Check sheet for the modelled part. Datum: model origin and axes. Units: mm. A direction names the side the tool comes from. Give positions to 0.01 mm unless a question says otherwise; leave off trailing zeros. Loops run counter-clockwise (first coordinate to the right, second up) from the corner with the lowest first, then second, coordinate; pieces in that order, holes last. Notation, with made-up numbers: (39.5, 12) -> (50.5, 12) arc R22 ccw to (50.5, 45) -> close; hole circle Ø2 at (32.25, 12). An arc over 180 degrees is marked (long way). Write each question's results on one line, items separated by ' | '. Start each with the question number.
1. Material ranges on L1, parallel to Z at x = 0, y = 29.5; L2, parallel to X at y = 36.5, z = -9.1; L3, parallel to Y at x = -0.35, z = -7.4, recorded low to high. Write a range as from..to.
2. Cross-section at B-B on y = 13. Record the boundary of the cut face in (x, z).
3. Gauge pin test, flat end, axial feed: pin 1 Ø0.8 at (x, z) = (0, -9) entering from -Y. Record the tip position at first contact, or that the pin passes through.
4. Tool access check on faces 5 (the face through (-0.011, 40.364, -5.496)), 6 (the face through (-0.104, 33.549, -9.793)). Record the directions out of +Z, -Z, +X, -X, +Y, -Y that give a thin tool (end or side, any length) a straight path to the whole face; none if there is none.
5. Cross-section at A-A on x = 0. Record the boundary of the cut face in (y, z), and give its area (3 significant figures).
6. Mould release check, pull along Y, two halves, no side actions. Record for faces 1 (the face through (-0.104, 12.591, -9.793)), 2 (the face through (0.43, 40.735, -6.483)), 3 (the face through (0.098, 24.423, -8.256)), 4 (the face through (-0.12, 2.96, -9.89)): +Y half, -Y half, draft (parallel to the pull), parting line (faces both ways), or undercut.
from build123d import *

# Parameters (mm, degrees)
SKETCH2_R         = 0.8
SKETCH4_R         = 0.9
EXTRUDE1_DEPTH    = 6
SKETCH5_OUTSIDE_W = 12.086
SKETCH5_OUTSIDE_H = 14.96
SKETCH5_OUTSIDE_R = 0.75
EXTRUDE3_DEPTH    = 11


with BuildPart() as part:
    # Sweep1: sweep along a path in Sketch1
    with BuildLine(Plane(origin=(0, 0, 0), x_dir=(0, 0, -1), z_dir=(1, 0, 0))) as sweep1_path:
        Line((9, 0), (9, 37))
        ThreePointArc((9, 37), (8.457456133, 38.720729309), (7.02606043, 39.819077862))
        Line((7.02606043, 39.819077862), (5.5, 40.374518435))
    # Sketch2 → Sweep1 (sweep)
    with BuildSketch(Plane(origin=(0, 0, 0), x_dir=(1, 0, 0), z_dir=(0, 1, 0))):
        with Locations((0, 9)):
            Circle(SKETCH2_R)
    sweep(path=sweep1_path.line)

    # Sketch4 → Extrude1 (add)
    with BuildSketch(Plane(origin=(0, 0, 0), x_dir=(1, 0, 0), z_dir=(0, 1, 0))):
        with Locations((0, 9)):
            Circle(SKETCH4_R)
    extrude(amount=EXTRUDE1_DEPTH)

    # Sketch5 outside → Extrude3 (cut)
    with BuildSketch(Plane(origin=(0, 19, 0), x_dir=(-1, 0, 0), z_dir=(0, 1, 0))):
        with Locations((0, -7.563)):
            Rectangle(SKETCH5_OUTSIDE_W, SKETCH5_OUTSIDE_H)
        with Locations((0, -9)):
            Circle(SKETCH5_OUTSIDE_R, mode=Mode.SUBTRACT)
    extrude(amount=EXTRUDE3_DEPTH, mode=Mode.SUBTRACT)


solid = part.part
Geometry says:
1) L1: -9.75..-8.25 | L2: -0.79..0.79 | L3: 38.8..40.45
2) outline: circle Ø1.6 at (0, -9)
3) pin 1: y = 0
4) face 5: +Z, +X, -X, +Y | face 6: none
5) outline: (0, -9.9) -> (6, -9.9) -> (6, -9.8) -> (19, -9.8) -> (19, -9.75) -> (30, -9.75) -> (30, -9.8) -> (37, -9.8) arc R3.8 ccw to (40.57, -7.3) -> (41.13, -5.77) -> (39.62, -5.23) -> (39.07, -6.75) arc R2.2 cw to (37, -8.2) -> (30, -8.2) -> (30, -8.25) -> (19, -8.25) -> (19, -8.2) -> (6, -8.2) -> (6, -8.1) -> (0, -8.1) -> close | area: 67.8 mm^2
6) face 1: undercut | face 2: parting line | face 3: undercut | face 4: draft
